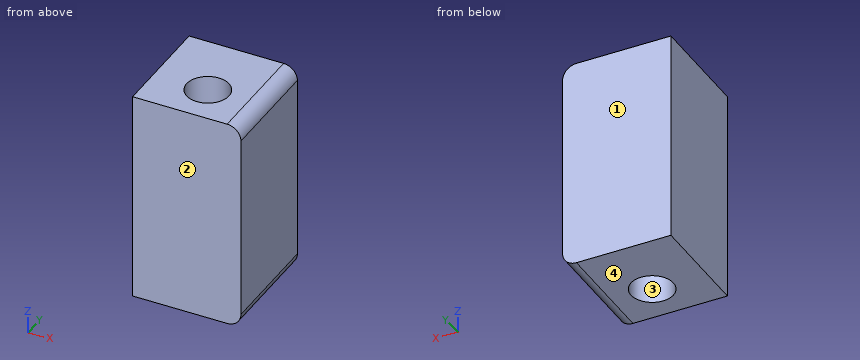
from build123d import *

# Parameters (mm, degrees)
SKETCH1_W           = 12.45
SKETCH1_H           = 24.5
BOSS_EXTRUDE1_DEPTH = 6.25
FILLET1_R           = 1.5875
SKETCH2_R           = 2.4384
CUT_EXTRUDE2_DEPTH  = 27.039645255


with BuildPart() as part:
    # Sketch1 → Boss-Extrude1 (new, symmetric)
    with BuildSketch(Plane(origin=(0, 0, 0), x_dir=(1, 0, 0), z_dir=(0, 1, 0))):
        Rectangle(SKETCH1_W, SKETCH1_H)
    extrude(amount=BOSS_EXTRUDE1_DEPTH, both=True)

    # Fillet1
    fillet1_edges = [part.edges().sort_by_distance(p)[0] for p in [
        (6.225, 0, 12.25),
        (6.225, 0, -12.25),
    ]]
    fillet(fillet1_edges, radius=FILLET1_R)

    # Sketch2 → Cut-Extrude2 (cut, through all)
    with BuildSketch(Plane(origin=(0, 0, -12.25), x_dir=(-1, 0, 0), z_dir=(0, 0, -1))):
        with Locations((0, -1.5875)):
            Circle(SKETCH2_R)
    extrude(amount=-CUT_EXTRUDE2_DEPTH, mode=Mode.SUBTRACT)


solid = part.part
Check sheet for the modelled part. Datum: model origin and axes. Units: mm. Face numbers are marked on the shaded views. Round coordinates to 2 decimals unless told otherwise and drop trailing zeros. Loops run counter-clockwise (first coordinate to the right, second up) from the corner with the lowest first, then second, coordinate; pieces in that order, holes last. Notation, with made-up numbers: M -26.75,24.25 L -4.75,24.25 A7 cw -4.75,30.25 Z; hole C -28,41 d2. An arc over 180 degrees is marked long. One line per item, written item: value.
(1) Release check for a two-part mould opening along Y. For the marked faces 1, 2, 3 and 4 record: +Y half, -Y half, draft (parallel to the pull), parting line (faces both ways), or undercut.
Computed values:
face 1: +Y half
face 2: -Y half
face 3: undercut
face 4: draft
(2) Thickness scan on line 1 (X direction, y = -1.75, z = 3) (3 decimals); line 2 (Y direction, x = 0, z = 5); line 3 (Y direction, x = 2, z = 0). Record the ranges inside material, lowest first.
Computed values:
line 1: x = -6.225 to -2.433, 2.433 to 6.225
line 2: y = -6.25 to -4.03, 0.85 to 6.25
line 3: y = -6.25 to -2.98, -0.19 to 6.25
(3) Sectioned sample at C-C, the plane x = -1.5. Record the cut outline in (y, z).
Computed values:
outline: M -6.25,-12.25 L -3.51,-12.25 L -3.51,12.25 L -6.25,12.25 Z; M 0.33,-12.25 L 6.25,-12.25 L 6.25,12.25 L 0.33,12.25 Z
(4) Sectioned sample at A-A, the plane x = 0. Record the cut outline in (y, z), then the cut area to 3 significant figures.
Computed values:
outline: M -6.25,-12.25 L -4.03,-12.25 L -4.03,12.25 L -6.25,12.25 Z; M 0.85,-12.25 L 6.25,-12.25 L 6.25,12.25 L 0.85,12.25 Z
area: 187 mm^2
